Answer from the drawing. Dimensions are ordinates in mm from the lowest x, y and z of the part. Round coordinates to 2 decimals unless told otherwise and drop trailing zeros. Loops run counter-clockwise (first coordinate to the right, second up) from the corner with the lowest first, then second, coordinate; pieces in that order, holes last. Notation, with made-up numbers: (52.25, 1) - (69.25, 1) arc R16 ccw to (69.25, 17) - close; hole circle Ø2 at (65.25, 61.25). An arc over 180 degrees is marked (long way). Use CSV: the item, a comma, the result in double quotes. Start each with the question number.
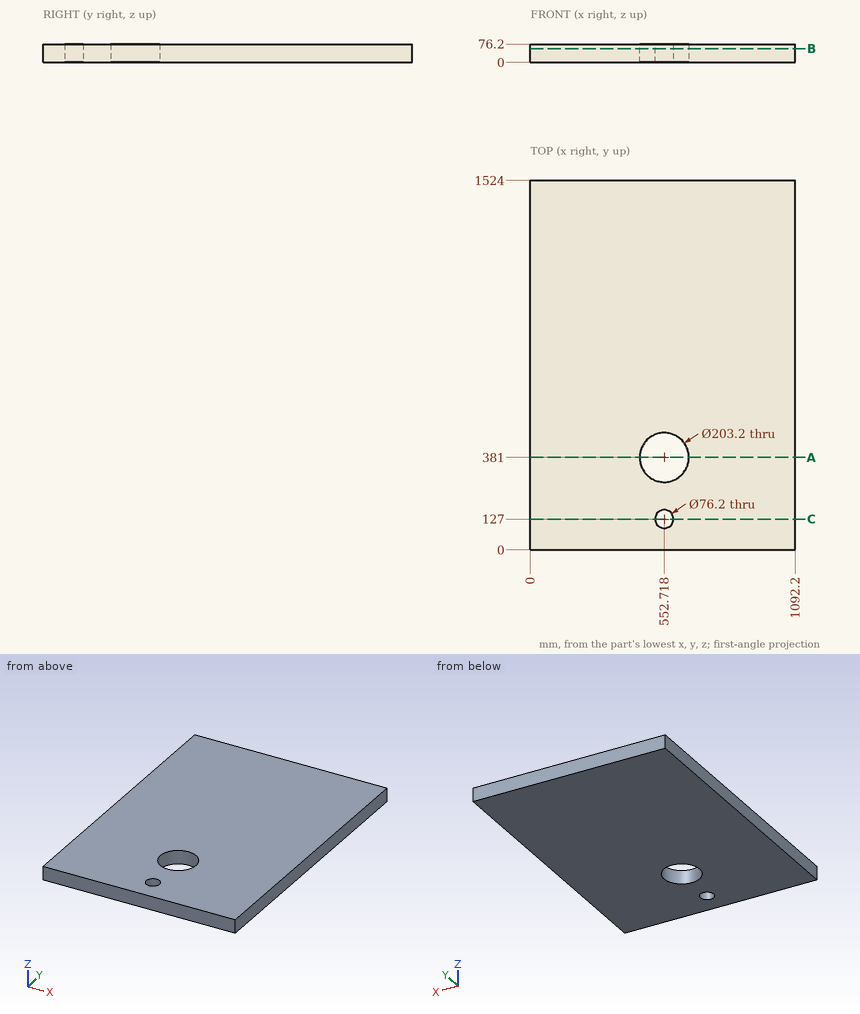
Item 1: A cutting plane is placed at A-A (y = 381). Determine the outline of the cut face in (x, z).
Item 2: Find the intervals of material crossed by probe 1 along X at (y, z) = (381, 24); probe 2 along Y at (x, z) = (572, 14); probe 3 along X at (y, z) = (127, 22), in increasing order. Write a range as [from, to].
Item 3: A cutting plane is placed at C-C (y = 127). Determine the outline of the cut face in (x, z).
Item 4: A cutting plane is placed at B-B (z = 57.5). Determine the outline of the cut face in (x, y).
Result sheet:
1,outline,"(0, 0) - (451.12, 0) - (451.12, 76.2) - (0, 76.2) - close; (654.32, 0) - (1092.2, 0) - (1092.2, 76.2) - (654.32, 76.2) - close"
2,probe 1,"[0, 451.12], [654.32, 1092.2]"
2,probe 2,"[0, 94.14], [159.86, 281.25], [480.75, 1524]"
2,probe 3,"[0, 514.62], [590.82, 1092.2]"
3,outline,"(0, 0) - (514.62, 0) - (514.62, 76.2) - (0, 76.2) - close; (590.82, 0) - (1092.2, 0) - (1092.2, 76.2) - (590.82, 76.2) - close"
4,outline,"(0, 0) - (1092.2, 0) - (1092.2, 1524) - (0, 1524) - close; hole circle Ø203.2 at (552.72, 381); hole circle Ø76.2 at (552.72, 127)"
